```python
from build123d import *

# Parameters (mm, degrees)
F1_DEPTH = 76.2
F2_SIZE  = 5.08
F3_SIZE  = 5.08
F4_R     = 5.08
F5_SIZE  = 5.08


with BuildPart() as f1:
    # F0 (on Front) → F1 (new body)
    with BuildSketch(Plane.XZ):
        Polygon((29.771948, -17.903628), (29.771948, 109.096372), (10.721948, 109.096372), (10.721948, 83.696372), (20.246948, 83.696372), (20.246948, 64.646372), (10.721948, 64.646372), (10.721948, -17.903628), align=None)
    extrude(amount=F1_DEPTH)

    # F2
    f2_edges = [f1.edges().sort_by_distance(p)[0] for p in [
        (29.771948, -38.1, 109.096372),
    ]]
    chamfer(f2_edges, length=F2_SIZE)

    # F3
    f3_edges = [f1.edges().sort_by_distance(p)[0] for p in [
        (17.706948, -76.2, 109.096372),
        (17.706948, 0, 109.096372),
    ]]
    chamfer(f3_edges, length=F3_SIZE)

    # F4
    f4_edges = [f1.edges().sort_by_distance(p)[0] for p in [
        (10.721948, -38.1, 109.096372),
    ]]
    fillet(f4_edges, radius=F4_R)

    # F5
    f5_edges = [f1.edges().sort_by_distance(p)[0] for p in [
        (10.721948, -76.2, 93.856372),
        (29.771948, -76.2, 43.056372),
        (10.721948, -76.2, 23.371372),
        (29.771948, 0, 43.056372),
        (10.721948, 0, 93.856372),
        (10.721948, 0, 23.371372),
    ]]
    chamfer(f5_edges, length=F5_SIZE)


solid = f1.part
```
Geometry: final body of the model. Coordinates: model frame, mm. A direction names the side the tool comes from. Round coordinates to 2 decimals unless told otherwise and drop trailing zeros. Order: outer loops, then holes, each group sorted by start corner. A loop starts at its lowest first (then second) coordinate and runs counter-clockwise, first axis right, second up. Notation, with made-up numbers: (78.25, -27) -> (132.25, -27) arc R18 cw to (132.25, -12) -> close; hole circle Ø4 at (25.25, 1.5). An arc over 180 degrees is marked (long way). Use one line per item in the form item = value.
(1) First-contact query: pin 1 Ø15 at (y, z) = (-38.5, 73) entering from -X; pin 2 Ø6 at (x, z) = (26, 73.5) entering from -Y. Flat tips, straight axial feed; report the tip coordinate or a pass-through.
Results list:
pin_1 = 20.25
pin_2 = -76.2
(2) Section A-A on z = 90. Return loops of the section in (x, y), and give its area (3 significant figures).
Results list:
outline = (10.72, -71.12) -> (15.8, -76.2) -> (24.69, -76.2) -> (29.77, -71.12) -> (29.77, -5.08) -> (24.69, 0) -> (15.8, 0) -> (10.72, -5.08) -> close
area = 1,400 mm^2
(3) Access query for faces 1 (the face through (20.247, -38, 74)), 2 (the face through (27.2, -37.6, 106.59)). Directions: +Z, -Z, +X, -X, +Y, -Y. A direction counts if a zero-diameter tool reaches every point of the face in a straight line with its end or side. Return the directions, or none.
Results list:
face_1 = -X, +Y, -Y
face_2 = +Z, +X, +Y, -Y
(4) Section C-C on y = -42.5. Return loops of the section in (x, z), and give its area (3 significant figures).
Results list:
outline = (10.72, -17.9) -> (29.77, -17.9) -> (29.77, 104.02) -> (24.69, 109.1) -> (15.8, 109.1) arc R5.08 ccw to (10.72, 104.02) -> (10.72, 83.7) -> (20.25, 83.7) -> (20.25, 64.65) -> (10.72, 64.65) -> close
area = 2,220 mm^2
(5) Draft query along Z for faces 3 (the face through (16, -38, 64.646)), 4 (the face through (19.826, -2.576, 106.592)), 5 (the face through (20, 0, 44)). Return one class per face: pulls with the +Z half, pulls with the -Z half, needs draft (parallel to the pull), parting line crosses it, or undercut.
Results list:
face_3 = undercut
face_4 = pulls with the +Z half
face_5 = needs draft
(6) Section B-B on x = 17. Return loops of the section in (y, z), and give its area (3 significant figures).
Results list:
outline = (-76.2, -17.9) -> (0, -17.9) -> (0, 64.65) -> (-76.2, 64.65) -> close; (-76.2, 83.7) -> (0, 83.7) -> (0, 104.02) -> (-5.08, 109.1) -> (-71.12, 109.1) -> (-76.2, 104.02) -> close
area = 8,200 mm^2
(7) Ray query, probe 1 along Z at (x, y) = (19, -22); probe 2 along X at (y, z) = (-7.5, 72); probe 3 along Z at (x, y) = (12.75, -40). Return the intervals inside material, ascending. Write a range as [from, to].
Results list:
probe_1 = [-17.9, 64.65], [83.7, 109.1]
probe_2 = [20.25, 29.77]
probe_3 = [-17.9, 64.65], [83.7, 108.08]
